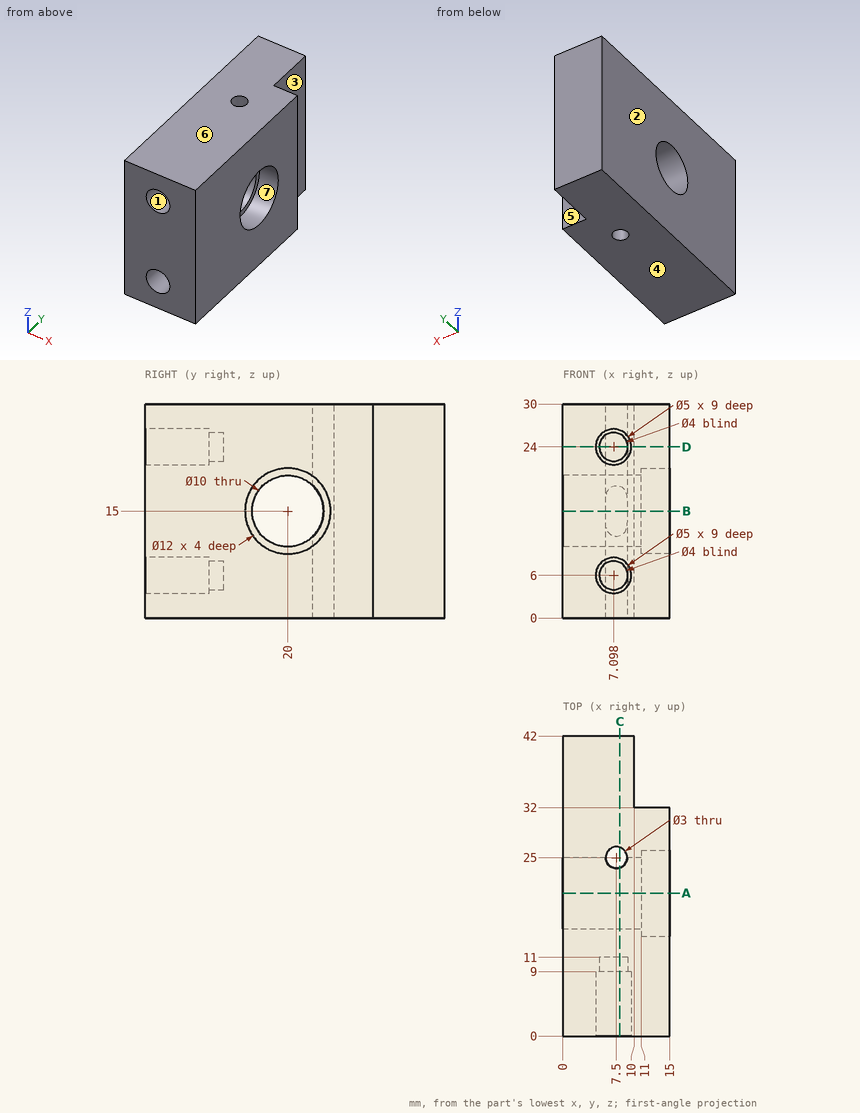
Can you work these out from the drawing? Everything is in mm from the part's minimum corner. A direction names the side the tool comes from. Give positions to 0.01 mm unless a question says otherwise; leave off trailing zeros. Order: outer loops, then holes, each group sorted by start corner. A loop starts at its lowest first (then second) coordinate and runs counter-clockwise, first axis right, second up. Notation, with made-up numbers: M 75.25,-22 L 80.25,-22 A21 ccw 80.25,-18 Z; hole C -13,62.5 d8. An arc over 180 degrees is marked long. Write item = value, one per line. Start each with the question number.
Q1. Will these pins go through, and if not, where does the flat tip stop? pin 1 Ø2.5 at (x, z) = (7.1, 24) entering from -Y; pin 2 Ø3 at (y, z) = (36.5, 11) entering from +X; pin 3 Ø4.5 at (x, z) = (7.1, 6) entering from -Y.
Q2. Suppose I cut it at A-A (y = 20). Write out the boundary of the cut face in (x, z), plus the area to 3 significant figures.
Q3. I need wall thicknesses on probe 1 along Z at (x, y) = (7, 8.5); probe 2 along X at (y, z) = (2, 24); probe 3 along X at (y, z) = (9.45, 6). Which ranges of each line are inside material? Lowest first, please. Write a range as [from, to].
Q4. Suppose I cut it at D-D (z = 24). Write out the boundary of the cut face in (x, y).
Q5. Suppose I cut it at C-C (x = 8). Write out the boundary of the cut face in (y, z) (1 decimal), plus the area to 3 significant figures.
Q6. Suppose I cut it at B-B (z = 15). Write out the boundary of the cut face in (x, y).
Q7. We'd pull the mould along Z, two halves only. Please class the marked faces 4, 5, 6 and 7: pulls with the +Z half, pulls with the -Z half, needs draft (parallel to the pull), parting line crosses it, or undercut.
Q8. For the marked faces 1, 2 and 3, which set-ups out of +Z, -Z, +X, -X, +Y, -Y let a thin tool reach every point of the face, with its end or its side?
Check result:
q1.pin_1 = 11
q1.pin_2 = 10
q1.pin_3 = 9
q2.outline = M 0,0 L 15,0 L 15,9 L 11,9 L 11,10 L 0,10 Z; M 0,20 L 11,20 L 11,21 L 15,21 L 15,30 L 0,30 Z
q2.area = 292 mm2
q3.probe_1 = [0, 3.5], [8.5, 21.5], [26.5, 30]
q3.probe_2 = [0, 4.6], [9.6, 15]
q3.probe_3 = [0, 5.1], [9.1, 15]
q4.outline = M 0,0 L 4.6,0 L 4.6,9 L 5.1,9 L 5.1,11 L 9.1,11 L 9.1,9 L 9.6,9 L 9.6,0 L 15,0 L 15,32 L 10,32 L 10,42 L 0,42 Z; hole C 7.5,25 d3
q5.outline = M 0,0 L 23.6,0 L 23.6,11.5 A5 cw long 23.6,18.5 L 23.6,30 L 0,30 L 0,26.3 L 9,26.3 L 9,25.8 L 11,25.8 L 11,22.2 L 9,22.2 L 9,21.7 L 0,21.7 L 0,8.3 L 9,8.3 L 9,7.8 L 11,7.8 L 11,4.2 L 9,4.2 L 9,3.7 L 0,3.7 Z; M 26.4,0 L 42,0 L 42,30 L 26.4,30 Z
q5.area = 1,010 mm2
q6.outline = M 0,0 L 15,0 L 15,14 L 11,14 L 11,15 L 0,15 Z; M 0,25 L 6,25 A1.5 cw 9,25 L 11,25 L 11,26 L 15,26 L 15,32 L 10,32 L 10,42 L 0,42 Z
q7.face_4 = pulls with the -Z half
q7.face_5 = needs draft
q7.face_6 = pulls with the +Z half
q7.face_7 = undercut
q8.face_1 = -Y
q8.face_2 = +Z, -Z, -X, +Y, -Y
q8.face_3 = +Z, -Z, +X, +Y
